CAD build for the part. Positions are in the model's coordinates, mm. Give positions to 0.01 mm unless a question says otherwise; leave off trailing zeros. Order: outer loops, then holes, each group sorted by start corner. A loop starts at its lowest first (then second) coordinate and runs counter-clockwise, first axis right, second up. Notation, with made-up numbers: (-11, -16.75) -> (-7, -16.75) arc R13 ccw to (-7, -0.75) -> close; hole circle Ø4 at (11, 72.5). An arc over 180 degrees is marked (long way). Use one line per item in the form item = value. Start each with the question number.
1) Cut at A-A, the plane x = 46.5. Give the cut face in (y, z), and give its area (3 significant figures).
2) Drop flat-ended pins along their axis: P1, Ø8, axis at x = 188.5, z = 1, coming from the -Y side; P2, Ø1.2, axis at y = 1.5, z = 13.5, coming from the +X side; P3, Ø1.5, axis at x = -81.5, y = -9, coming from the -Z side; P4, Ø1, axis at x = -238.5, z = 12.5, coming from the -Y side. Give the stop position or say it passes through.
3) Probe line 1 (Y direction, x = 53, z = 1.5); line 2 (Z direction, x = 174, y = 9); line 3 (Y direction, x = 172.5, z = 6.25). List the from-to ranges inside material, lowest first.
4) Mould opens along Y. For faces 1 (the face through (-250, 0, 0)), 2 (the face through (230, 0, 11.157)), 3 (the face through (-230, 0, 11.157)), 4 (the face through (-249.81, -0.49, -12.18)) say: pulls with the +Y half, pulls with the -Y half, needs draft (parallel to the pull), parting line crosses it, or undercut.
from build123d import *

# Parameters (mm, degrees)
F0_W     = 500
F0_H     = 15
F3_DEPTH = 40
F4_SIZE2 = 3
F4_SIZE  = 3


# Not quite as in the source:
# - a pattern or mirror of a feature is missing from the dataset's text; its kind, count and spacing are read off the source's solid


with BuildPart() as f1:
    # F0 (on Top) → F1 (revolve)
    with BuildSketch(Plane.XY):
        with Locations((0, 7.5)):
            Rectangle(F0_W, F0_H)
    revolve(axis=Axis((0, 0, 0), (1, 0, 0)))

    # F2 (on face) → F3 (cut)
    with BuildSketch(Plane.YZ.offset(250)):
        with BuildLine():
            ThreePointArc((4, 14.4568322948), (0, 15), (-4, 14.4568322948))
            Line((-4, 14.4568322948), (-4, 11.1568322948))
            Line((-4, 11.1568322948), (4, 11.1568322948))
            Line((4, 11.1568322948), (4, 14.4568322948))
        make_face()
    f3 = extrude(amount=-F3_DEPTH, mode=Mode.SUBTRACT)

    # F3_copies: F3 across plane
    add(f3.mirror(Plane(origin=(0, 0, 0), x_dir=(0, 0, -1), z_dir=(-1, 0, 0))), mode=Mode.SUBTRACT)

    # F4
    f4_edges = [f1.edges().sort_by_distance(p)[0] for p in [
        (250, -9.082951, -11.937336),
        (250, 11.937336, 9.082951),
        (-250, 11.937336, 9.082951),
        (-250, -9.082951, -11.937336),
    ]]
    chamfer(f4_edges, length=F4_SIZE, length2=F4_SIZE2)


solid = f1.part
Result:
q1.outline = circle Ø30 at (0, 0)
q1.area = 707 mm²
q2.P1 = -15
q2.P2 = 210
q2.P3 = -12.53
q2.P4 = -9
q3.line_1 = -14.92 to 14.92
q3.line_2 = -12 to 12
q3.line_3 = -13.64 to 13.64
q4.face_1 = needs draft
q4.face_2 = undercut
q4.face_3 = undercut
q4.face_4 = parting line crosses it
